from build123d import *

# Parameters (mm, degrees)
EXTRUDE_1_DEPTH = 12
SKETCH_1_3_R    = 7
SKETCH_1_3_R_2  = 3
EXTRUDE_2_DEPTH = 3
EXTRUDE_START   = 9
SKETCH_1_4_R    = 7
SKETCH_1_4_R_2  = 3
EXTRUDE_3_DEPTH = 3
FILLET_1_R      = 1


with BuildPart() as part:
    # 草图1 → 凸台-拉伸1 (new body)
    with BuildSketch(Plane(origin=(0, 0, 0), x_dir=(1, 0, 0), z_dir=(0, 1, 0))):
        with BuildLine():
            add(Edge.make_bspline(
                [(-3.908610404, 5.807130506), (-12.380011049, 3.605621884), (-27.376579438, 6.317559199), (-39.425413051, 17.773045339), (-45.658717555, 24.846396214), (-47.987295244, 26.48198888)],
                knots=[0, 0, 0, 0, 0.514096191, 0.795654463, 1, 1, 1, 1], degree=3))
            Line((-47.987295244, 26.48198888), (-49.136854466, 24.845372371))
            add(Edge.make_bspline(
                [(-49.136854466, 24.845372371), (-44.808882779, 21.086502798), (-40.758819083, 14.514483032), (-28.442702771, 1.362936195), (-15.62875807, -2.307960271), (-5.630384559, -4.159178971)],
                knots=[0, 0, 0, 0, 0.315330411, 0.428800605, 1, 1, 1, 1], degree=3))
            ThreePointArc((-5.630384559, -4.159178971), (-6.897821205, 1.191663806), (-3.908610404, 5.807130506))
        make_face()
    extrude(amount=EXTRUDE_1_DEPTH)

    # 草图1<3> → 凸台-拉伸2 (add)
    with BuildSketch(Plane(origin=(0, 0, 0), x_dir=(1, 0, 0), z_dir=(0, 1, 0))):
        Circle(SKETCH_1_3_R)
        with Locations(Location((-0.421324482, -0.852481629, 0), (0, 0, 270))):
            Circle(SKETCH_1_3_R_2, mode=Mode.SUBTRACT)
    extrude(amount=EXTRUDE_2_DEPTH)

    # 草图1<4> → 凸台-拉伸3 (add)
    with BuildSketch(Plane(origin=(0, 0, 0), x_dir=(1, 0, 0), z_dir=(0, 1, 0)).offset(EXTRUDE_START)):
        Circle(SKETCH_1_4_R)
        with Locations(Location((-0.421324482, -0.852481629, 0), (0, 0, 270))):
            Circle(SKETCH_1_4_R_2, mode=Mode.SUBTRACT)
    extrude(amount=EXTRUDE_3_DEPTH)

    # 圆角1
    fillet_1_edges = [part.edges().sort_by_distance(p)[0] for p in [
        (-47.987295244, 6, -26.48198888),
        (-48.562074855, 0, -25.663680626),
        (-48.562074855, 12, -25.663680626),
        (-49.136854466, 6, -24.845372371),
    ]]
    fillet(fillet_1_edges, radius=FILLET_1_R)


solid = part.part
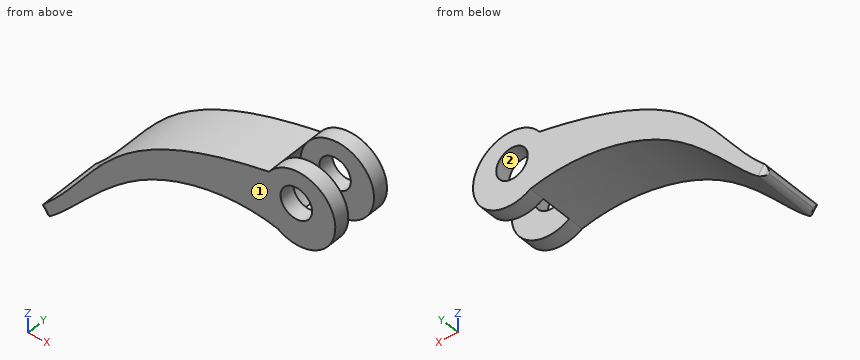
The listing builds one solid part. Answer for the finished solid, in the listing's coordinates (mm). Face numbers are marked on the shaded views. Give positions to 0.01 mm unless a question says otherwise; leave off trailing zeros.
1) Find the intervals of material crossed by L1, parallel to Y at x = -0.5, z = -5; L2, parallel to X at y = 11.25, z = -16; L3, parallel to Z at x = 1, y = 9.5, in increasing order.
2) Section A-A (z = 3) is taken. Count the separate pieces of the cut face and the enclosed holes in it, and give its area (3 significant figures).
3) For a pull along X with two mould halves and no side action, classify the marked faces 1 and 2 as pulls with the +X half, pulls with the -X half, needs draft (parallel to the pull), parting line crosses it, or undercut.
4) Given P1, Ø5, axis at x = -13.5, y = 10.5, coming from the +Z side; P2, Ø4, axis at x = -26.5, y = 8, coming from the -Z side; P3, Ø4, axis at x = -29, y = 2.5, coming from the -Z side; P4, Ø5, axis at x = -0.42, z = 0.85, coming from the +Y side, each flat-ended and moving along its own axis, determine where each tip first touches the part or whether it passes through.
Response:
1. L1: y = 0 to 3, 9 to 12
1. L2: x = -41.41 to -37.38
1. L3: z = -6.93 to -1.79, 3.49 to 6.93
2. separate pieces: 3
2. enclosed holes: 0
2. area: 109 mm2
3. face 1: needs draft
3. face 2: undercut
4. P1: stops at z = 3.04
4. P2: stops at z = -9.21
4. P3: stops at z = -10.73
4. P4: passes through
